Check sheet for the modelled part. Datum: model origin and axes. Units: mm. Round coordinates to 2 decimals unless told otherwise and drop trailing zeros. Order: outer loops, then holes, each group sorted by start corner. A loop starts at its lowest first (then second) coordinate and runs counter-clockwise, first axis right, second up. Notation, with made-up numbers: (14, 13) -> (52, 13) arc R35 cw to (52, 48) -> close; hole circle Ø8 at (65, 41.5). An arc over 180 degrees is marked (long way). Answer in a Markdown table with one row per item. Add a question column.
1. Material ranges on L1, parallel to X at y = 179.5, z = 1.5; L2, parallel to Y at x = 181, z = 1.9, recorded low to high. Write a range as from..to.
2. Sectioned sample at D-D, the plane y = 192.25. Record the boundary of the cut face in (x, z), then the cut area to 3 significant figures.
3. Sectioned sample at C-C, the plane x = 164. Record the boundary of the cut face in (y, z), then the cut area to 3 significant figures.
4. Sectioned sample at A-A, the plane x = 78.25. Count the separate pieces of the cut face and the enclosed holes in it, then the cut area to 4 significant figures.
Autodesk Inventor part; units mm, degrees
ref_plane "YZ Plane" through (0, 0, 0) normal (1, 0, 0) x (0, 1, 0)
ref_plane "XZ Plane" through (0, 0, 0) normal (0, 1, 0) x (-1, 0, 0)
ref_plane "XY Plane" through (0, 0, 0) normal (0, 0, 1) x (1, 0, 0)
sketch "Sketch1" plane through (0, 0, 0) normal (0, 0, 1) x (1, 0, 0)
  line L0 (0, 0) -> (214, 0)
  line L1 (214, 0) -> (214, 214)
  line L2 (214, 214) -> (0, 214)
  line L3 (0, 214) -> (0, 0)
  dimension "d0" = 214
  dimension "d1" = 214
extrude "Extrusion1" add sketch "Sketch1" along normal blind 3
sketch "Sketch2" plane through (0, 0, 3) normal (0, 0, 1) x (1, 0, 0)
  line L0 (207, 207) -> (7, 207)
  line L1 (7, 207) -> (7, 7)
  line L2 (7, 7) -> (207, 7)
  line L3 (207, 7) -> (207, 207)
  line L4 (207, 207) -> (7, 7) construction
  line L5 (7, 207) -> (207, 7) construction
  line L6 (7, 7) -> (35.5, 7)
  line L7 (35.5, 7) -> (35.5, 35.5)
  line L8 (35.5, 35.5) -> (7, 35.5)
  line L9 (7, 35.5) -> (7, 7)
  circle A0 centre (21.25, 21.25) radius 10.25
  point P0 (0, 0)
  point P1 (107, 107)
  dimension "d4" = 200
  dimension "d5" = 200
  dimension "d6" = 28.5
  dimension "d7" = 28.5
  dimension "d8" = 20.5
extrude "Extrusion2" cut sketch "Sketch2" against normal blind 3 contours A0
pattern_linear "Rectangular Pattern1" count 7 spacing 28.5 along (1, 0, 0) count 5 spacing 28.5 along (0, 1, 0) of "Extrusion2"
sketch "Sketch3" plane through (0, 0, 3) normal (0, 0, 1) x (1, 0, 0)
  circle A0 centre (21.25, 135.25) radius 10.25
  line L0 (21.25, 135.25) -> (21.25, 163.75)
  circle A1 centre (21.25, 163.75) radius 10.25
  point P0 (0, 0)
  dimension "d17" = 28.5
  dimension "d18" = 20.5
extrude "Extrusion3" cut sketch "Sketch3" against normal blind 3 contours A1
pattern_linear "Rectangular Pattern2" count 5 spacing 28.5 along (1, 0, 0) count 2 spacing 28.5 along (0, 1, 0) of "Extrusion3"
sketch "Sketch4" plane through (0, 0, 3) normal (0, 0, 1) x (1, 0, 0)
  line L0 (7, 7) -> (207, 7)
  line L1 (207, 7) -> (207, 207)
  line L2 (207, 207) -> (7, 207)
  line L3 (7, 207) -> (7, 7)
  line L4 (7, 7) -> (207, 207) construction
  line L5 (207, 7) -> (7, 207) construction
  line L6 (207, 207) -> (152, 207)
  line L7 (152, 207) -> (152, 152)
  line L8 (152, 152) -> (207, 152)
  line L9 (207, 152) -> (207, 207)
  circle A0 centre (179.5, 179.5) radius 27.5
  point P0 (0, 0)
  point P1 (107, 107)
  dimension "d27" = 200
  dimension "d28" = 200
  dimension "d29" = 55
  dimension "d30" = 55
extrude "Extrusion4" cut sketch "Sketch4" against normal blind 3 contours A0
properties part number "inert indsats plade"
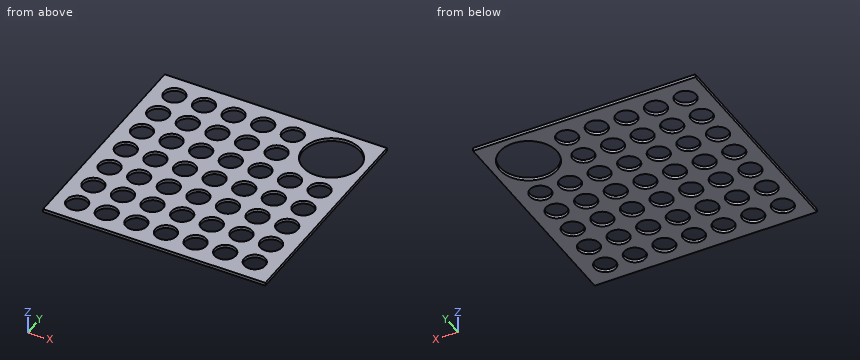
Answer key:
| question | item | result |
|---|---|---|
| 1 | L1 | x = 0..152, 207..214 |
| 1 | L2 | y = 0..152.04, 206.96..214 |
| 2 | outline | (0, 0) -> (11, 0) -> (11, 3) -> (0, 3) -> close; (31.5, 0) -> (39.5, 0) -> (39.5, 3) -> (31.5, 3) -> close; (60, 0) -> (68, 0) -> (68, 3) -> (60, 3) -> close; (88.5, 0) -> (96.5, 0) -> (96.5, 3) -> (88.5, 3) -> close; (117, 0) -> (125, 0) -> (125, 3) -> (117, 3) -> close; (145.5, 0) -> (155.13, 0) -> (155.13, 3) -> (145.5, 3) -> close; (203.87, 0) -> (214, 0) -> (214, 3) -> (203.87, 3) -> close |
| 2 | area | 188 mm² |
| 3 | outline | (0, 0) -> (11, 0) -> (11, 3) -> (0, 3) -> close; (31.5, 0) -> (39.5, 0) -> (39.5, 3) -> (31.5, 3) -> close; (60, 0) -> (68, 0) -> (68, 3) -> (60, 3) -> close; (88.5, 0) -> (96.5, 0) -> (96.5, 3) -> (88.5, 3) -> close; (117, 0) -> (125, 0) -> (125, 3) -> (117, 3) -> close; (145.5, 0) -> (156.78, 0) -> (156.78, 3) -> (145.5, 3) -> close; (202.22, 0) -> (214, 0) -> (214, 3) -> (202.22, 3) -> close |
| 3 | area | 198 mm² |
| 4 | separate pieces | 8 |
| 4 | enclosed holes | 0 |
| 4 | area | 211.5 mm² |
